Input: part model. Units: mm. Frame: model coordinates. Coordinates: 2 decimals unless noted, no trailing zeros. Answer in a Markdown table with one row per item.
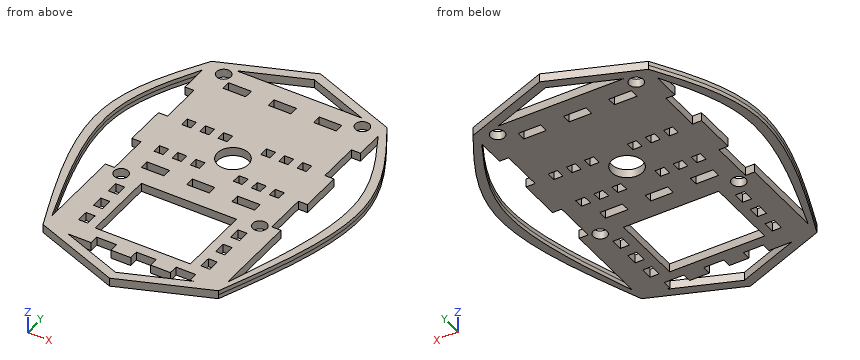
from build123d import *

# Parameters (mm, degrees)
F0_W     = 3.2
F0_H     = 4.2
F0_R     = 2.5
F0_W_2   = 8
F0_H_2   = 3.2
F0_W_3   = 33.5989631712
F0_H_3   = 26.0656554639
F0_R_2   = 5.5
F1_DEPTH = 1.5


with BuildPart() as f1:
    # F0 (on Top) → F1 (new body, symmetric)
    with BuildSketch(Plane.XY):
        with BuildLine():
            Line((0, -69.8), (31, -57.8))
            add(Edge.make_bspline(
                [(31, 37.5), (38.1511552694, 25.7567925156), (53.9932959403, -0.2582411241), (39.1454927008, -37.415537584), (31, -57.8)],
                knots=[0, 0, 0, 0, 0.4514008187, 1, 1, 1, 1], degree=3))
            Line((31, 37.5), (0, 49.5))
            Line((0, 49.5), (-31, 37.5))
            add(Edge.make_bspline(
                [(-31, 37.5), (-38.1511552694, 25.7567925156), (-53.9932959403, -0.2582411241), (-39.1454927008, -37.415537584), (-31, -57.8)],
                knots=[0, 0, 0, 0, 0.4514008187, 1, 1, 1, 1], degree=3))
            Line((-31, -57.8), (0, -69.8))
        make_face()
        with Locations((-21.6, -48.02561)):
            Rectangle(F0_W, F0_H, mode=Mode.SUBTRACT)
        with Locations((-21.6, -39.62561)):
            Rectangle(F0_W, F0_H, mode=Mode.SUBTRACT)
        with Locations((-21.6, -31.22561)):
            Rectangle(F0_W, F0_H, mode=Mode.SUBTRACT)
        with Locations((-24.5, -24)):
            Circle(F0_R, mode=Mode.SUBTRACT)
        with Locations((-17, -16.6)):
            Rectangle(F0_W_2, F0_H_2, mode=Mode.SUBTRACT)
        with Locations((-1, -16.6)):
            Rectangle(F0_W_2, F0_H_2, mode=Mode.SUBTRACT)
        Polygon((0, -66.37), (-22.14, -57.8), (-14, -57.8), (-14, -54.6), (-7, -54.6), (-7, -57.8), (0, -57.8), (0, -54.6), (7, -54.6), (7, -57.8), (14, -57.8), (14, -54.6), (21, -54.6), (21, -57.8), (22.14, -57.8), align=None, mode=Mode.SUBTRACT)
        with Locations((21.6, -48.02561)):
            Rectangle(F0_W, F0_H, mode=Mode.SUBTRACT)
        with Locations((0, -37.95)):
            Rectangle(F0_W_3, F0_H_3, mode=Mode.SUBTRACT)
        with Locations((21.6, -39.62561)):
            Rectangle(F0_W, F0_H, mode=Mode.SUBTRACT)
        with Locations((21.6, -31.22561)):
            Rectangle(F0_W, F0_H, mode=Mode.SUBTRACT)
        with Locations((24.5, -24)):
            Circle(F0_R, mode=Mode.SUBTRACT)
        with Locations((15, -16.6)):
            Rectangle(F0_W_2, F0_H_2, mode=Mode.SUBTRACT)
        with BuildLine():
            Line((-31, -22.5), (-31, -32.5))
            Line((-31, -32.5), (-31, -52.8))
            add(Edge.make_bspline(
                [(-31, 32.5), (-36.5997895584, 22.3876839263), (-49.2002368333, -0.3666899989), (-37.5003288582, -34.0731141218), (-31, -52.8)],
                knots=[0, 0, 0, 0, 0.444411967, 1, 1, 1, 1], degree=3))
            Line((-31, 32.5), (-31, 22.5))
            Line((-31, 22.5), (-27.8, 22.5))
            Line((-27.8, 22.5), (-27.8, 7.5))
            Line((-27.8, 7.5), (-31, 7.5))
            Line((-31, 7.5), (-31, -7.5))
            Line((-31, -7.5), (-27.8, -7.5))
            Line((-27.8, -7.5), (-27.8, -22.5))
            Line((-27.8, -22.5), (-31, -22.5))
        make_face(mode=Mode.SUBTRACT)
        with Locations((-20.4, -7.8)):
            Rectangle(F0_W, F0_H_2, mode=Mode.SUBTRACT)
        with Locations((-14, -7.8)):
            Rectangle(F0_W, F0_H_2, mode=Mode.SUBTRACT)
        with Locations((-7.6, -7.8)):
            Rectangle(F0_W, F0_H_2, mode=Mode.SUBTRACT)
        with Locations((-20.4, 7.8)):
            Rectangle(F0_W, F0_H_2, mode=Mode.SUBTRACT)
        with Locations((-14, 7.8)):
            Rectangle(F0_W, F0_H_2, mode=Mode.SUBTRACT)
        with Locations((-7.6, 7.8)):
            Rectangle(F0_W, F0_H_2, mode=Mode.SUBTRACT)
        with Locations((-24.5, 34)):
            Circle(F0_R, mode=Mode.SUBTRACT)
        with Locations((-17, 29.6)):
            Rectangle(F0_W_2, F0_H_2, mode=Mode.SUBTRACT)
        with Locations((-1, 29.6)):
            Rectangle(F0_W_2, F0_H_2, mode=Mode.SUBTRACT)
        Polygon((22.1355892594, 37.5), (0, 37.5), (-22.1355892594, 37.5), (0, 46.0686151972), align=None, mode=Mode.SUBTRACT)
        with Locations((7.6, -7.8)):
            Rectangle(F0_W, F0_H_2, mode=Mode.SUBTRACT)
        Circle(F0_R_2, mode=Mode.SUBTRACT)
        with Locations((14, -7.8)):
            Rectangle(F0_W, F0_H_2, mode=Mode.SUBTRACT)
        with Locations((20.4, -7.8)):
            Rectangle(F0_W, F0_H_2, mode=Mode.SUBTRACT)
        with Locations((7.6, 7.8)):
            Rectangle(F0_W, F0_H_2, mode=Mode.SUBTRACT)
        with Locations((14, 7.8)):
            Rectangle(F0_W, F0_H_2, mode=Mode.SUBTRACT)
        with Locations((20.4, 7.8)):
            Rectangle(F0_W, F0_H_2, mode=Mode.SUBTRACT)
        with BuildLine():
            Line((27.8, 7.5), (27.8, 22.5))
            Line((27.8, 22.5), (31, 22.5))
            Line((31, 22.5), (31, 32.5))
            add(Edge.make_bspline(
                [(31, 32.5), (36.5997895584, 22.3876839263), (49.2002368333, -0.3666899989), (37.5003288582, -34.0731141218), (31, -52.8)],
                knots=[0, 0, 0, 0, 0.444411967, 1, 1, 1, 1], degree=3))
            Line((31, -52.8), (31, -32.5))
            Line((31, -32.5), (31, -22.5))
            Line((31, -22.5), (27.8, -22.5))
            Line((27.8, -22.5), (27.8, -7.5))
            Line((27.8, -7.5), (31, -7.5))
            Line((31, -7.5), (31, 7.5))
            Line((31, 7.5), (27.8, 7.5))
        make_face(mode=Mode.SUBTRACT)
        with Locations((15, 29.6)):
            Rectangle(F0_W_2, F0_H_2, mode=Mode.SUBTRACT)
        with Locations((24.5, 34)):
            Circle(F0_R, mode=Mode.SUBTRACT)
    extrude(amount=F1_DEPTH, both=True)


solid = f1.part
1) Contact query for flat-ended pins moving along their axis: pin 1 (4.5 mm diameter, centred on x = -24.5, y = 34, fed in from +Z); pin 2 (0.9 mm diameter, centred on y = 8, z = 0, fed in from -X); pin 3 (1.5 mm diameter, centred on x = -7.5, z = -0.5, fed in from +Y); pin 4 (1 mm diameter, centred on x = -25.5, z = 0, fed in from -Y). Output: stop coordinate, or through.
Resolved:
| item | result |
|---|---|
| pin 1 | passes through |
| pin 2 | stops at x = -45.1 |
| pin 3 | stops at y = 46.89 |
| pin 4 | stops at y = -60.12 |
2) Cut plane A-A, the plane z = 0.5. State how many separate pieces and enclosed holes the cut face has, and give its area (3 significant figures).
Resolved:
| item | result |
|---|---|
| separate pieces | 1 |
| enclosed holes | 34 |
| area | 5,140 mm2 |
3) Material intervals for probe 1 along Y at (x, z) = (-24.5, 0.2); probe 2 along X at (y, z) = (-23, -1.1); probe 3 along Y at (x, z) = (4.5, 0.35), sorted ascending.
Resolved:
| item | result |
|---|---|
| probe 1 | y = -60.32 to -26.5, -21.5 to 31.5, 36.5 to 40.02 |
| probe 2 | x = -43.37 to -40.35, -31 to -26.79, -22.21 to 22.21, 26.79 to 31, 40.35 to 43.37 |
| probe 3 | y = -68.06 to -64.63, -54.6 to -50.98, -24.92 to -3.16, 3.16 to 37.5, 44.33 to 47.76 |
